Check sheet for the modelled part. Datum: model origin and axes. Units: mm. A direction names the side the tool comes from. Coordinates: 2 decimals unless noted, no trailing zeros. Loops run counter-clockwise (first coordinate to the right, second up) from the corner with the lowest first, then second, coordinate; pieces in that order, holes last. Notation, with made-up numbers: (43.5, 48.25) - (59.5, 48.25) arc R30 ccw to (59.5, 81.25) - close; hole circle Ø6 at (52.25, 29.25). An arc over 180 degrees is marked (long way). Use a Markdown table: item, result. Add a question column.
1) Thickness scan on line 1 (X direction, y = -54, z = 0); line 2 (X direction, y = 70.5, z = 29); line 3 (Z direction, x = 176, y = 24.5). Record the ranges inside material, lowest first.
2) Sectioned sample at C-C, the plane y = 151. Enter the section's corners in (x, z), then the cut area to 3 significant figures.
3) Go/stop test with flat-tipped pins: P1, Ø10.5, axis at y = -166.5, z = -50, coming from the +X side; P2, Ø1.5, axis at x = -17, z = -19, coming from the +Y side; P3, Ø8, axis at x = 82.5, z = 3.5, coming from the -Y side; P4, Ø10.5, axis at y = -143.5, z = -52, coming from the -X side. Record where each tip stops, or that it passes through.
4) Sectioned sample at A-A, the plane x = -86. Enter the section's corners in (y, z), then the cut area to 3 significant figures.
5) Tool access check on faces 1 (the flat face through (252.168, -81.165, -18)), 2 (the flat face through (-252.17, 87.98, 43.56)), 3 (the flat face through (251.83, 87.98, 43.56)). Record the directions out of +Z, -Z, +X, -X, +Y, -Y that give a thin tool (end or side, any length) a straight path to the whole face; none if there is none.
6) Sectioned sample at D-D, the plane x = -171.5. Enter the section's corners in (y, z), then the cut area to 3 significant figures.
7) Sectioned sample at B-B, the plane x = 98.5. Enter the section's corners in (y, z), then the cut area to 3 significant figures.
from build123d import *

# Parameters (mm, degrees)
F2_R     = 110
F3_DEPTH = 22


with BuildPart() as f3:
    # F2 (on face) → F3 (new body)
    with BuildSketch(Plane(origin=(0, 0, 0), x_dir=(1, 0, 0), z_dir=(0, 0.34202, -0.939693))):
        Polygon((-194, 183), (-194, 139), (-240, 122.426697), (-240, 82.426697), (-264, 82.426697), (-264, -97.573303), (-240, -97.573303), (-219.132979, -183), (-160, -183), (160, -183), (219.132978, -183), (240, -97.573303), (264, -97.573303), (264, 82.426697), (240, 82.426697), (240, 122.426697), (194, 139), (194, 183), align=None)
        with Locations((0, -7.573303)):
            Circle(F2_R, mode=Mode.SUBTRACT)
    extrude(amount=-F3_DEPTH)


solid = f3.part
Solved:
| question | item | result |
|---|---|---|
| 1 | line 1 | x = -264 to -93.27, 93.27 to 264 |
| 1 | line 2 | x = -264 to -85.99, 85.99 to 264 |
| 1 | line 3 | z = 8.92 to 32.33 |
| 2 | outline | (-224.58, 54.96) - (224.58, 54.96) - (222.63, 78.37) - (-222.63, 78.37) - close |
| 2 | area | 10,500 mm2 |
| 3 | P1 | stops at x = 194 |
| 3 | P2 | stops at y = -100.38 |
| 3 | P3 | passes through |
| 3 | P4 | stops at x = -194 |
| 4 | outline | (-179.49, -41.92) - (-171.96, -62.59) - (-57.33, -20.87) - (-64.86, -0.19) - close; (64.04, 46.72) - (71.57, 26.05) - (171.96, 62.59) - (164.44, 83.26) - close |
| 4 | area | 5,030 mm2 |
| 5 | face 1 | -Z, +X, -Y |
| 5 | face 2 | +Z, -X, +Y |
| 5 | face 3 | +Z, +X, +Y |
| 6 | outline | (-179.49, -41.92) - (-171.96, -62.59) - (171.96, 62.59) - (164.44, 83.26) - close |
| 6 | area | 8,050 mm2 |
| 7 | outline | (-179.49, -41.92) - (-171.96, -62.59) - (-38.9, -14.16) - (-46.42, 6.52) - close; (45.61, 40.01) - (53.13, 19.34) - (171.96, 62.59) - (164.44, 83.26) - close |
| 7 | area | 5,900 mm2 |
